Input: part model. Units: mm. Frame: model coordinates. A direction names the side the tool comes from. Coordinates: 2 decimals unless noted, no trailing zeros. Loops run counter-clockwise (first coordinate to the right, second up) from the corner with the lowest first, then second, coordinate; pieces in that order, holes last. Notation, with made-up numbers: (-26.75, -32) -> (5.25, -32) arc R22 ccw to (5.25, -21) -> close; hole circle Ø10 at (-16, -8). An arc over 180 degrees is marked (long way). Answer as a JSON object with one key per item and string values.
from build123d import *

# Parameters (mm, degrees)
BOSS_EXTRUDE1_DEPTH = 15
FILLET1_R           = 7.5
CHAMFER1_SIZE       = 5
SKETCH2_R           = 2.2
CUT_EXTRUDE1_DEPTH  = 10
SKETCH3_W           = 12
SKETCH3_H           = 2
BOSS_EXTRUDE2_DEPTH = 3.8
SKETCH4_W           = 12
SKETCH4_H           = 8
BOSS_EXTRUDE3_DEPTH = 5
FILLET2_R           = 3
BOSS_EXTRUDE4_DEPTH = 12


with BuildPart() as part:
    # Sketch1 → Boss-Extrude1 (new body)
    with BuildSketch(Plane(origin=(0, 0, 0), x_dir=(1, 0, 0), z_dir=(0, 1, 0))):
        with BuildLine():
            Line((7.5, 27), (122.5, 27))
            ThreePointArc((122.5, 27), (127.803300859, 24.803300859), (130, 19.5))
            Line((130, 19.5), (130, 7.5))
            ThreePointArc((130, 7.5), (127.803300859, 2.196699141), (122.5, 0))
            Line((122.5, 0), (7.5, 0))
            ThreePointArc((7.5, 0), (2.196699141, 2.196699141), (0, 7.5))
            Line((0, 7.5), (0, 19.5))
            ThreePointArc((0, 19.5), (2.196699141, 24.803300859), (7.5, 27))
        make_face()
    extrude(amount=BOSS_EXTRUDE1_DEPTH)

    # Fillet1
    fillet1_edges = [part.edges().sort_by_distance(p)[0] for p in [
        (0, 0, -13.5),
        (2.196699141, 0, -24.803300859),
        (65, 0, -27),
        (127.803300859, 0, -24.803300859),
        (130, 0, -13.5),
        (127.803300859, 0, -2.196699141),
        (65, 0, 0),
        (2.196699141, 0, -2.196699141),
    ]]
    fillet(fillet1_edges, radius=FILLET1_R)

    # Chamfer1
    # the kernel refuses this chamfer: 5 mm, written as the material it takes off along each edge
    with BuildSketch(Plane(origin=(0, 15, 5.35841494), x_dir=(-0.02749587661058638, -0.9996219169112968, 0), z_dir=(0, 0, -1))) as chamfer1_piece_1:
        Polygon((CHAMFER1_SIZE * 0.999621916911, -CHAMFER1_SIZE * 0.0274958766106), (-CHAMFER1_SIZE * 0.0274958766106, -CHAMFER1_SIZE * 0.999621916911), (0, 0), align=None)
    extrude(amount=37.71682988, mode=Mode.SUBTRACT)

    # Sketch2 → Cut-Extrude1 (cut)
    with BuildSketch(Plane(origin=(0, 15, 0), x_dir=(1, 0, 0), z_dir=(0, 1, 0))):
        with Locations(Location((5, 22, 0), (0, 0, 270))):
            Circle(SKETCH2_R)
        with Locations(Location((5, 5, 0), (0, 0, 270))):
            Circle(SKETCH2_R)
    extrude(amount=-CUT_EXTRUDE1_DEPTH, mode=Mode.SUBTRACT)

    # Sketch3 → Boss-Extrude2 (add)
    with BuildSketch(Plane(origin=(0, 15, 0), x_dir=(1, 0, 0), z_dir=(0, 1, 0))):
        with Locations((101, 21)):
            Rectangle(SKETCH3_W, SKETCH3_H)
    extrude(amount=BOSS_EXTRUDE2_DEPTH)

    # Sketch4 → Boss-Extrude3 (add)
    with BuildSketch(Plane(origin=(0, 18.8, 0), x_dir=(1, 0, 0), z_dir=(0, 1, 0))):
        with Locations((101, 18)):
            Rectangle(SKETCH4_W, SKETCH4_H)
    extrude(amount=BOSS_EXTRUDE3_DEPTH)

    # Fillet2
    fillet2_edges = [part.edges().sort_by_distance(p)[0] for p in [
        (101, 23.8, -22),
    ]]
    fillet(fillet2_edges, radius=FILLET2_R)

    # Sketch5 → Boss-Extrude4 (add)
    with BuildSketch(Plane.ZY.offset(-95)):
        Polygon((-20, 18.8), (-17, 18.8), (-20, 16.9), align=None)
    extrude(amount=-BOSS_EXTRUDE4_DEPTH)


solid = part.part
1. Line query: line 1 along Z through (x, y) = (5, 9.25); line 2 along Y through (x, z) = (89, -10.75); line 3 along X through (y, z) = (10, -22). Output: solid intervals per line, ascending.
Reply:
{"line 1": "z = -26.57 to -24.2, -19.8 to -7.2, -2.8 to -0.43", "line 2": "y = 0 to 15", "line 3": "x = 0.43 to 2.8, 7.2 to 129.57"}
2. Section query C-C (z = -8.75). Return loops of the section in (x, y).
Reply:
{"outline": "(0, 7.5) arc R7.5 ccw to (7.5, 0) -> (122.5, 0) arc R7.5 ccw to (130, 7.5) -> (130, 15) -> (5, 15) -> (0, 10) -> close"}
3. Mould query, pull axis X, two halves, no side actions, for faces 1 (the face through (127.861, 2.255, -13.416)), 2 (the face through (101, 21, -14)), 3 (the face through (5, 5, -5)). Classes: pulls with the +X half, pulls with the -X half, needs draft (parallel to the pull), parting line crosses it, or undercut.
Reply:
{"face 1": "pulls with the +X half", "face 2": "needs draft", "face 3": "undercut"}
4. Access query for faces 4 (the face through (7.18, 10.07, -5.29)), 5 (the face through (64, 11, -27)), 6 (the face through (107, 20, -18)). Directions: +Z, -Z, +X, -X, +Y, -Y. A direction counts if a zero-diameter tool reaches every point of the face in a straight line with its end or side. Return the directions, or none.
Reply:
{"face 4": "+Y", "face 5": "-Z, +X, -X, +Y, -Y", "face 6": "+Z, -Z, +X, +Y"}
5. Section query B-B (x = 60.5). Return loops of the section in (y, z), plus the area to 3 significant figures.
Reply:
{"outline": "(0, -19.5) arc R7.5 ccw to (7.5, -27) -> (15, -27) -> (15, 0) -> (7.5, 0) arc R7.5 ccw to (0, -7.5) -> close", "area": "381 mm2"}
6. Section query A-A (y = 1.5). Return loops of the section in (x, z), plus the area to 3 significant figures.
Reply:
{"outline": "(3, -19.5) arc R4.5 ccw to (7.5, -24) -> (122.5, -24) arc R4.5 ccw to (127, -19.5) -> (127, -7.5) arc R4.5 ccw to (122.5, -3) -> (7.5, -3) arc R4.5 ccw to (3, -7.5) -> close", "area": "2,590 mm2"}
7. Pin query (flat end, axial travel): P1, Ø5.5, axis at x = 101, y = 22, coming from the +Z side; P2, Ø3, axis at y = 13.5, z = -19.5, coming from the -X side; P3, Ø1.3, axis at x = 5.5, z = -4.5, coming from the +Y side; P4, Ø12, axis at x = 27.5, y = 20, coming from the -Z side. Return the tip coordinate at first contact, or that it passes through.
Reply:
{"P1": "stops at z = -14", "P2": "stops at x = 2", "P3": "stops at y = 5", "P4": "stops at z = -27"}
